```python
from build123d import *

# Parameters (mm, degrees)
SKETCH1_R           = 11.2
SKETCH1_R_2         = 1.75
BOSS_EXTRUDE1_DEPTH = 5
BOSS_EXTRUDE2_DEPTH = 25
CUT_EXTRUDE1_DEPTH  = 77.661594035
SKETCH4_R           = 2.7
CUT_EXTRUDE2_DEPTH  = 25
FILLET1_R           = 1
BOSS_EXTRUDE3_DEPTH = 5
BOSS_EXTRUDE4_DEPTH = 5


with BuildPart() as part:
    # Sketch1 → Boss-Extrude1 (new body)
    with BuildSketch(Plane.XY):
        with BuildLine():
            Line((26.5, 34), (-26.5, 34))
            Line((-26.5, 34), (-26.5, 26.7))
            Line((-26.5, 26.7), (-20, 26.7))
            ThreePointArc((-20, 26.7), (-17.3, 24), (-20, 21.3))
            Line((-20, 21.3), (-26.5, 21.3))
            Line((-26.5, 21.3), (-26.5, -34))
            Line((-26.5, -34), (26.5, -34))
            Line((26.5, -34), (26.5, 21.3))
            Line((26.5, 21.3), (20, 21.3))
            ThreePointArc((20, 21.3), (17.3, 24), (20, 26.7))
            Line((20, 26.7), (26.5, 26.7))
            Line((26.5, 26.7), (26.5, 34))
        make_face()
        with Locations((0, -13)):
            Circle(SKETCH1_R, mode=Mode.SUBTRACT)
        with Locations((15.5, 2.5)):
            Circle(SKETCH1_R_2, mode=Mode.SUBTRACT)
        with Locations(Location((15.5, -28.5, 0), (0, 0, 180))):
            Circle(SKETCH1_R_2, mode=Mode.SUBTRACT)
        with Locations(Location((-15.5, 2.5, 0), (0, 0, 180))):
            Circle(SKETCH1_R_2, mode=Mode.SUBTRACT)
        with Locations((-15.5, -28.5)):
            Circle(SKETCH1_R_2, mode=Mode.SUBTRACT)
    extrude(amount=BOSS_EXTRUDE1_DEPTH)

    # Sketch2 → Boss-Extrude2 (add)
    with BuildSketch(Plane(origin=(0, 0, 0), x_dir=(-1, 0, 0), z_dir=(0, 0, -1))):
        Polygon((26.5, -34), (21.5, -34), (21.5, 9), (37.5, 9), (37.5, 4), (26.5, 4), align=None)
        Polygon((-26.5, 4), (-26.5, -34), (-21.5, -34), (-21.5, 9), (-37.5, 9), (-37.5, 4), align=None)
    extrude(amount=BOSS_EXTRUDE2_DEPTH)

    # Sketch3 → Cut-Extrude1 (cut, through all)
    with BuildSketch(Plane.ZY.offset(26.5)):
        Polygon((-25, 4), (0, -34), (-25, -34), align=None)
    extrude(amount=-CUT_EXTRUDE1_DEPTH, mode=Mode.SUBTRACT)

    # Sketch4 → Cut-Extrude2 (cut)
    with BuildSketch(Plane.XZ.offset(-4)):
        with Locations((32, -15)):
            Circle(SKETCH4_R)
        with Locations(Location((-32, -15, 0), (0, 0, 270))):
            Circle(SKETCH4_R)
    extrude(amount=-CUT_EXTRUDE2_DEPTH, mode=Mode.SUBTRACT)

    # Fillet1
    fillet1_edges = [part.edges().sort_by_distance(p)[0] for p in [
        (-26.5, 21.3, 2.5),
        (-26.5, 26.7, 2.5),
        (26.5, 21.3, 2.5),
        (26.5, 26.7, 2.5),
        (26.5, 34, 2.5),
        (26.5, -34, 2.5),
        (-26.5, -34, 2.5),
        (-26.5, 34, 2.5),
        (-37.5, 4, -12.5),
        (-37.5, 9, -12.5),
        (-21.5, 9, -12.5),
        (21.5, 9, -12.5),
        (37.5, 4, -12.5),
        (37.5, 9, -12.5),
    ]]
    fillet(fillet1_edges, radius=FILLET1_R)

    # Sketch5 → Boss-Extrude3 (add)
    with BuildSketch(Plane.XY):
        with BuildLine():
            Line((26.5, 4), (36.5, 4))
            ThreePointArc((36.5, 4), (37.207106781, 4.292893219), (37.5, 5))
            Line((37.5, 5), (37.5, 8))
            ThreePointArc((37.5, 8), (37.207106781, 8.707106781), (36.5, 9))
            Line((36.5, 9), (26.5, 9))
            Line((26.5, 9), (26.5, 4))
        make_face()
    extrude(amount=BOSS_EXTRUDE3_DEPTH)

    # Sketch6 → Boss-Extrude4 (add)
    with BuildSketch(Plane.XY):
        with BuildLine():
            Line((-37.5, 8), (-37.5, 5))
            ThreePointArc((-37.5, 5), (-37.207106781, 4.292893219), (-36.5, 4))
            Line((-36.5, 4), (-26.5, 4))
            Line((-26.5, 4), (-26.5, 9))
            Line((-26.5, 9), (-36.5, 9))
            ThreePointArc((-36.5, 9), (-37.207106781, 8.707106781), (-37.5, 8))
        make_face()
    extrude(amount=BOSS_EXTRUDE4_DEPTH)


solid = part.part
```
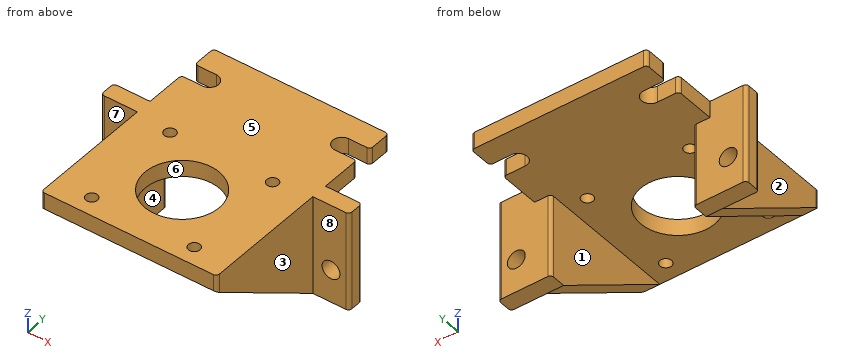
Here's how the part is built. I have some questions about the finished solid (model axes, mm). Face numbers are marked on the shaded views. A direction names the side the tool comes from. Coordinates: 2 decimals unless noted, no trailing zeros. Loops run counter-clockwise (first coordinate to the right, second up) from the corner with the lowest first, then second, coordinate; pieces in that order, holes last. Notation, with made-up numbers: M 40.5,-2 L 84.5,-2 A16 ccw 84.5,20 Z; hole C 2,59.25 d6. An arc over 180 degrees is marked long. One line per item, written item: value.
1. Imagine slicing it at B-B (x = -15.5). List the corners of the cut face in (y, z) for me.
Geometry says:
outline: M -34,0 L -30.25,0 L -30.25,5 L -34,5 Z; M -26.75,0 L 0.75,0 L 0.75,5 L -26.75,5 Z; M 4.25,0 L 34,0 L 34,5 L 4.25,5 Z
2. Will these pins go through, and if not, where does the flat tip stop? pin 1 Ø5.5 at (x, y) = (15.5, 2.5) entering from -Z; pin 2 Ø3 at (y, z) = (-9.5, -12.5) entering from -X; pin 3 Ø4 at (x, z) = (27, -7) entering from +Y.
Geometry says:
pin 1: stops at z = 0
pin 2: stops at x = -26.5
pin 3: stops at y = 9
3. Imagine slicing it at A-A (z = -19). List the corners of the cut face in (x, y) for me, and give its area (3 significant figures).
Geometry says:
outline: M -37.5,5 A1 ccw -36.5,4 L -26.5,4 L -26.5,-5.12 L -21.5,-5.12 L -21.5,8 A1 ccw -22.5,9 L -36.5,9 A1 ccw -37.5,8 Z; M 21.5,-5.12 L 26.5,-5.12 L 26.5,4 L 36.5,4 A1 ccw 37.5,5 L 37.5,8 A1 ccw 36.5,9 L 22.5,9 A1 ccw 21.5,8 Z
area: 250 mm2
4. Please list where these lines run through material, in increasing order: probe 1 along Y at (x, z) = (15.5, 2.65); probe 2 along X at (y, z) = (-15.5, -8.5); probe 3 along Z at (x, y) = (-18.5, -23).
Geometry says:
probe 1: y = -34 to -30.25, -26.75 to 0.75, 4.25 to 34
probe 2: x = -26.5 to -21.5, 21.5 to 26.5
probe 3: z = 0 to 5
5. Imagine slicing it at D-D (y = -28.5). List the corners of the cut face in (x, z) for me, and give its area (3 significant figures).
Geometry says:
outline: M -26.5,-3.62 L -21.5,-3.62 L -21.5,0 L -17.25,0 L -17.25,5 L -26.5,5 Z; M -13.75,0 L 13.75,0 L 13.75,5 L -13.75,5 Z; M 17.25,0 L 21.5,0 L 21.5,-3.62 L 26.5,-3.62 L 26.5,5 L 17.25,5 Z
area: 266 mm2
6. On a 3-axis mill with a long thin cutter (end or side, diameter ignored), from which of +Z, -Z, +X, -X, +Y, -Y can I reach the whole of each face in a straight line? I mean the marked faces 4, 5, 6, 7 and 8. Say none if no direction works.
Geometry says:
face 4: -Z, +Y, -Y
face 5: +Z, +X, -X, +Y, -Y
face 6: +Z, -Z
face 7: +Z, -Z, -X, -Y
face 8: +Z, -Z, +X, -Y
7. Imagine slicing it at C-C (z = -15). List the corners of the cut face in (x, y) for me.
Geometry says:
outline: M -37.5,5 A1 ccw -36.5,4 L -34.7,4 L -34.7,9 L -36.5,9 A1 ccw -37.5,8 Z; M -29.3,4 L -26.5,4 L -26.5,-11.2 L -21.5,-11.2 L -21.5,8 A1 ccw -22.5,9 L -29.3,9 Z; M 21.5,-11.2 L 26.5,-11.2 L 26.5,4 L 29.3,4 L 29.3,9 L 22.5,9 A1 ccw 21.5,8 Z; M 34.7,4 L 36.5,4 A1 ccw 37.5,5 L 37.5,8 A1 ccw 36.5,9 L 34.7,9 Z
8. Thinking about a two-plate mould opening in X: for the marked faces 1, 2 and 3, which applies, +X half, -X half, draft (parallel to the pull), parting line (faces both ways), or undercut?
Geometry says:
face 1: undercut
face 2: -X half
face 3: +X half
